CAD build for the part. Positions are in the model's coordinates, mm. Face numbers are marked on the shaded views. A direction names the side the tool comes from. Coordinates: 2 decimals unless noted, no trailing zeros. Order: outer loops, then holes, each group sorted by start corner. A loop starts at its lowest first (then second) coordinate and runs counter-clockwise, first axis right, second up. Notation, with made-up numbers: M 8,0 L 66,0 A27 ccw 66,20 Z; hole C -3,46 d7. An arc over 180 degrees is marked long. One line per item, written item: value.
from build123d import *

# Parameters (mm, degrees)
SKETCH2_R          = 57.049339495
CUT_EXTRUDE1_DEPTH = 5


with BuildPart() as part:
    # Sketch1 → Revolve1 (revolve)
    with BuildSketch(Plane.XY, mode=Mode.PRIVATE) as revolve1_sk:
        Polygon((0, 0), (75.266699621, 0), (106.605503378, 65.757917285), (93.480705223, 65.757917285), (68.367246776, 13.062583534), (0, 13.062583534), align=None)
    revolve(revolve1_sk.sketch.rotate(Axis((0, 73.257801944, 0), (0, -1, 0)), 90), axis=Axis((0, 73.257801944, 0), (0, -1, 0)))

    # Sketch2 → Cut-Extrude1 (cut)
    with BuildSketch(Plane(origin=(0, 13.062583534, 0), x_dir=(1, 0, 0), z_dir=(0, 1, 0))):
        with Locations(Location((0, 0, 0), (0, 0, 270))):
            Circle(SKETCH2_R)
    extrude(amount=-CUT_EXTRUDE1_DEPTH, mode=Mode.SUBTRACT)


solid = part.part
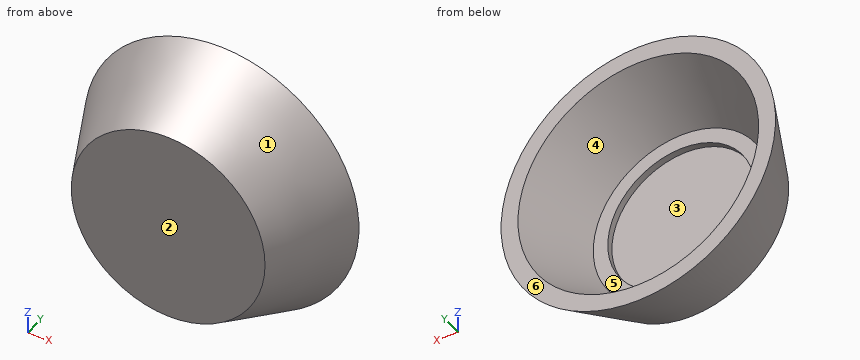
Q1. Drill centre lines: line 1 along Y through (x, z) = (-3.5, -40); line 2 along Z through (x, y) = (-64, 36.5); line 3 along Z through (x, y) = (39, 40). Where is each one in solid material? Low to high.
Recorded:
line 1: y = 0 to 8.06
line 2: z = -67.01 to -47.22, 47.22 to 67.01
line 3: z = -85.89 to -71.23, 71.23 to 85.89
Q2. Pin check, flat tips, straight feed: pin 1 Ø2 at (y, z) = (58.5, 45.5) entering from +X; pin 2 Ø3 at (x, y) = (-77.5, 58.5) entering from +Z; pin 3 Ø5 at (y, z) = (17, -53.5) entering from -X. Stop position of each tip, or through.
Recorded:
pin 1: stops at x = 93.29
pin 2: stops at z = 70.05
pin 3: stops at x = -66.47
Q3. Slice it at C-C (y = 48). List the corners of the cut face in (x, z).
Recorded:
outline: C 0,0 d196.28; hole C 0,0 d170.04
Q4. Which spindle directions (+Z, -Z, +X, -X, +Y, -Y) get a long thin tool onto all of the face, cutting with end or side? Do the marked faces 5 and 6. Say none if no direction does.
Recorded:
face 5: +Y
face 6: +Z, -Z, +X, -X, +Y
Q5. Slice it at A-A (z = 0). List the corners of the cut face in (x, y).
Recorded:
outline: M -106.61,65.76 L -75.27,0 L 75.27,0 L 106.61,65.76 L 93.48,65.76 L 68.37,13.06 L 57.05,13.06 L 57.05,8.06 L -57.05,8.06 L -57.05,13.06 L -68.37,13.06 L -93.48,65.76 Z
Q6. Mould opens along Z. For the marked faces 1, 2, 3 and 4 say: released by +Z, released by -Z, zero draft, split by the parting line, or undercut.
Recorded:
face 1: split by the parting line
face 2: zero draft
face 3: undercut
face 4: undercut
Q7. Slice it at B-B (x = 0). List the corners of the cut face in (y, z), plus the area to 3 significant figures.
Recorded:
outline: M 0,-75.27 L 65.76,-106.61 L 65.76,-93.48 L 13.06,-68.37 L 13.06,-57.05 L 8.06,-57.05 L 8.06,57.05 L 13.06,57.05 L 13.06,68.37 L 65.76,93.48 L 65.76,106.61 L 0,75.27 Z
area: 2,860 mm^2
